from build123d import *

# Parameters (mm, degrees)
F0_R          = 10
F1_DEPTH      = 150
F2_R          = 9.75
F3_DEPTH      = 153.7
F3_DEPTH_BACK = 18.1


with BuildPart() as f1:
    # F0 (on Top) → F1 (new body)
    with BuildSketch(Plane.XY):
        Circle(F0_R)
    extrude(amount=F1_DEPTH)

    # F2 (on Top) → F3 (join, two sides)
    with BuildSketch(Plane.XY) as f3_sk:
        Circle(F2_R)
    extrude(amount=F3_DEPTH)
    extrude(f3_sk.sketch, amount=-F3_DEPTH_BACK)


solid = f1.part
Build history of the part. All positions in model axes, mm. A direction names the side the tool comes from. Coordinates: 2 decimals unless noted, no trailing zeros. Order: outer loops, then holes, each group sorted by start corner. A loop starts at its lowest first (then second) coordinate and runs counter-clockwise, first axis right, second up. Notation, with made-up numbers: (54.5, -12.75) - (98.5, -12.75) arc R11 ccw to (98.5, -5.75) - close; hole circle Ø4 at (50.25, 82.25). An arc over 180 degrees is marked (long way). Write item = value, one per line. Start each with the question number.
1) Saw through at A-A on x = -2.75. Write the cut outline in (y, z), then the cut area to 3 significant figures.
2) Flat gauge pins, fed straight in: pin 1 Ø1 at (y, z) = (-5.5, 60.5) entering from +X; pin 2 Ø3 at (x, z) = (8, 0) entering from -Y; pin 3 Ø8 at (y, z) = (6.5, 68.5) entering from +X. Where does each tip first touch, or does it go through?
3) Wall check: line 1 along Y through (x, z) = (-2.25, 42); line 2 along Y through (x, z) = (-0.75, 35); line 3 along X through (y, z) = (-5.5, 81.5). Give the ranges that are in metal, low to high. Write a range as from..to.
4) Saw through at C-C on z = 125.5. Write the cut outline in (x, y).
5) 3-axis set-ups, long thin cutter, end or side, ignore diameter. For faces 1 (the face through (0, 0, 153.7)), 2 (the face through (-1.269, 9.667, 151.824)), 3 (the face through (-1.269, 9.667, -8.923)): which of +Z, -Z, +X, -X, +Y, -Y reach the whole face in a straight line?
6) Saw through at B-B on y = 3. Write the cut outline in (x, z), then the cut area to 3 significant figures.
From the geometry:
q1.outline = (-9.61, 0) - (-9.35, 0) - (-9.35, -18.1) - (9.35, -18.1) - (9.35, 0) - (9.61, 0) - (9.61, 150) - (9.35, 150) - (9.35, 153.7) - (-9.35, 153.7) - (-9.35, 150) - (-9.61, 150) - close
q1.area = 3,290 mm^2
q2.pin_1 = 8.66
q2.pin_2 = -7.6
q2.pin_3 = 9.68
q3.line_1 = -9.74..9.74
q3.line_2 = -9.97..9.97
q3.line_3 = -8.35..8.35
q4.outline = circle Ø20 at (0, 0)
q5.face_1 = +Z, +X, -X, +Y, -Y
q5.face_2 = +Z
q5.face_3 = -Z
q6.outline = (-9.54, 0) - (-9.28, 0) - (-9.28, -18.1) - (9.28, -18.1) - (9.28, 0) - (9.54, 0) - (9.54, 150) - (9.28, 150) - (9.28, 153.7) - (-9.28, 153.7) - (-9.28, 150) - (-9.54, 150) - close
q6.area = 3,270 mm^2
